Can you work these out from the model? Positions are in its coordinate system, mm. Face numbers are marked on the shaded views. A direction names the side the tool comes from. Give positions to 0.01 mm unless a question says otherwise; leave off trailing zeros. Order: outer loops, then holes, each group sorted by start corner. A loop starts at its lowest first (then second) coordinate and runs counter-clockwise, first axis right, second up. Notation, with made-up numbers: (26.5, 32.5) -> (73.5, 32.5) arc R17 cw to (73.5, 60.5) -> close; hole circle Ø10 at (6, -35). An arc over 180 degrees is marked (long way). Answer as CSV lines item,"result".
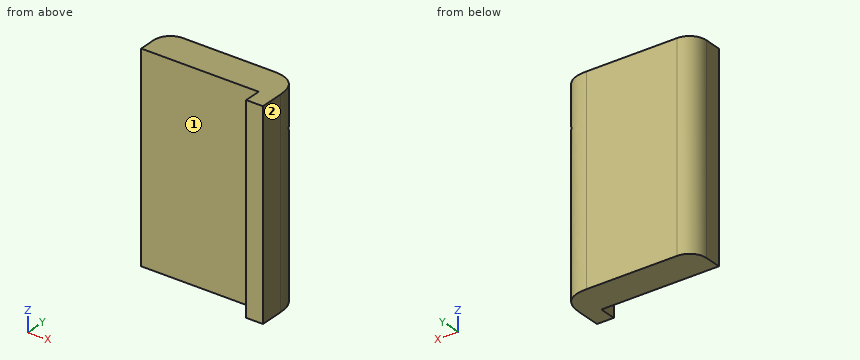
```python
from build123d import *

# Parameters (mm, degrees)
F0_W        = 40
F0_H        = 15
F1_DEPTH    = 60
F2_W        = 35
F2_H        = 5
F3_DEPTH    = 60
F4_T1_DEPTH = 100
F5_R        = 5


# Not quite as in the source:
# - a fillet or chamfer that OpenCascade refuses, or shapes differently, is made with other operations: its cross-section is extruded or revolved along the edge and cut away or added


with BuildPart() as f1:
    # F0 (on Top) → F1 (new body)
    with BuildSketch(Plane.XY):
        with Locations((20, -7.5)):
            Rectangle(F0_W, F0_H)
    extrude(amount=F1_DEPTH)

    # F2 (on face) → F3 (cut, through all)
    with BuildSketch(Plane.XY.offset(60)):
        with Locations((17.5, -12.5)):
            Rectangle(F2_W, F2_H)
    extrude(amount=-F3_DEPTH, mode=Mode.SUBTRACT)

    # F4: fillet of radius 8 on 1 edges, made by hand

    # F4_s2 → F4_t1 (cut)
    with BuildSketch(Plane.XY.offset(-20)):
        with BuildLine():
            add(Edge.make_bspline(
                [(32, 0), (40, 0), (40, -8)],
                knots=[0, 0, 0, 1, 1, 1], degree=2, weights=[1, 1, 1]))
            Line((40, -8), (40, 0))
            Line((40, 0), (32, 0))
        make_face()
    extrude(amount=F4_T1_DEPTH, mode=Mode.SUBTRACT)

    # F5
    f5_edges = [f1.edges().sort_by_distance(p)[0] for p in [
        (0, 0, 30),
    ]]
    fillet(f5_edges, radius=F5_R)


solid = f1.part
```
Item 1: Please list where these lines run through material, in increasing order: line 1 along Y through (x, z) = (5, 52.5); line 2 along X through (y, z) = (-11.75, 9.5); line 3 along X through (y, z) = (-2, 30.5).
Numbers:
line 1,"y = -10 to 0"
line 2,"x = 35 to 40"
line 3,"x = 1 to 38"
Item 2: Imagine slicing it at A-A, the plane y = -13.5. Please give me the cut outline in (x, z).
Numbers:
outline,"(35, 0) -> (40, 0) -> (40, 60) -> (35, 60) -> close"
Item 3: For the marked faces 1 and 2, which set-ups out of +Z, -Z, +X, -X, +Y, -Y let a thin tool reach every point of the face, with its end or its side?
Numbers:
face 1,"+Z, -Z, -X, -Y"
face 2,"+Z, -Z, +X, +Y, -Y"
Item 4: Imagine slicing it at B-B, the plane x = 21. Please give me the cut outline in (y, z), then the cut area to 3 significant figures.
Numbers:
outline,"(-10, 0) -> (0, 0) -> (0, 60) -> (-10, 60) -> close"
area,"600 mm²"
Item 5: For pin 1 (12 mm diameter, centred on x = 31.5, z = 22.5, fed in from -Y); pin 2 (3 mm diameter, centred on x = 18, z = 24.5, fed in from -Y), each with a flat end and sliding along its axis, tell me the tip position at first contact or that it passes through.
Numbers:
pin 1,"stops at y = -15"
pin 2,"stops at y = -10"
